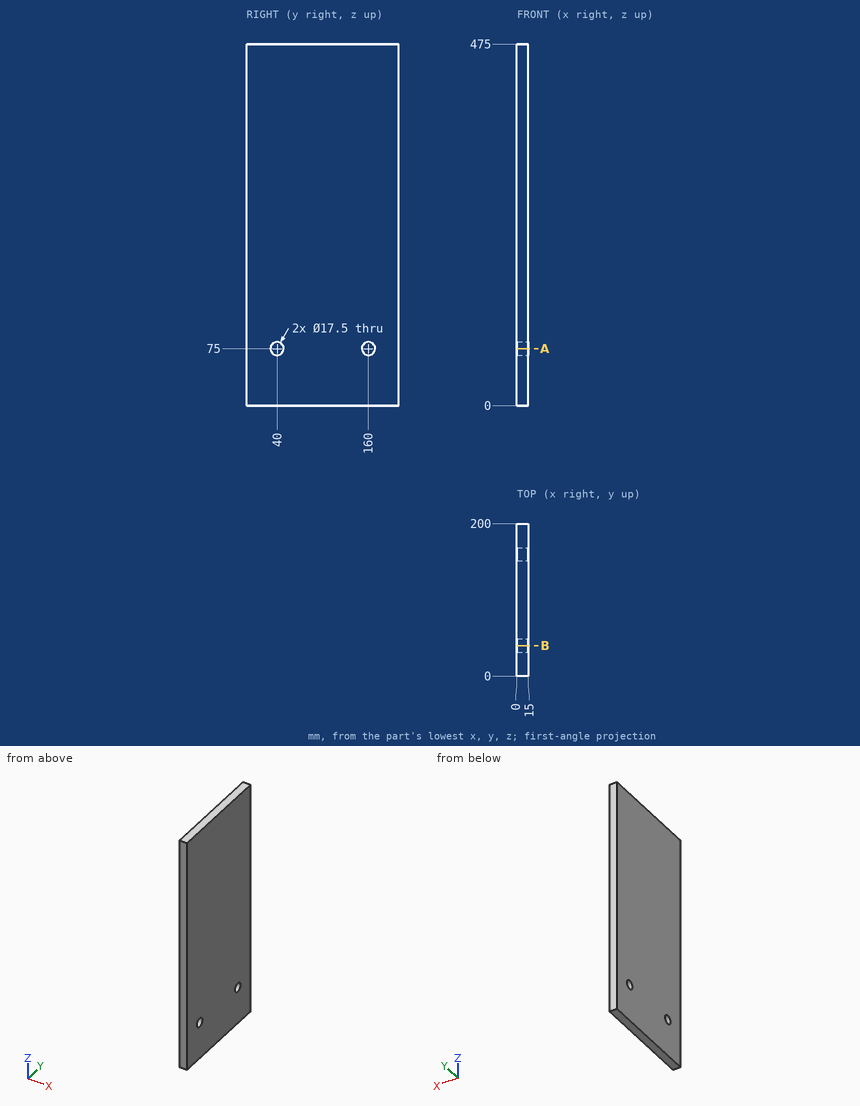
Geometry check sheet. Reference: drawing and pictorial views, mm from the part's lowest x, y, z. Give positions to 0.01 mm unless a question says otherwise; leave off trailing zeros. Write each loop counter-clockwise with the first axis right and the second up, starting at its lowest first coordinate (ties: lowest second). Pieces come first, ordered by that corner, then holes. Notation, with made-up numbers: (-11, -37.5) -> (26, -37.5) arc R11 ccw to (26, -29.5) -> close; hole circle Ø1 at (51, 74). An arc over 180 degrees is marked (long way). One line per question, with ' | ' between items.
Item 1: Sectioned sample at A-A, the plane z = 75. Record the boundary of the cut face in (x, y).
Determined:
outline: (0, 0) -> (15, 0) -> (15, 31.25) -> (0, 31.25) -> close; (0, 48.75) -> (15, 48.75) -> (15, 151.25) -> (0, 151.25) -> close; (0, 168.75) -> (15, 168.75) -> (15, 200) -> (0, 200) -> close
Item 2: Scan lines: line 1 along Z through (x, y) = (7, 160); line 2 along Y through (x, z) = (9.5, 75); line 3 along Z through (x, y) = (3.75, 32). Record each from-to range of solid material in increasing order.
Determined:
line 1: 0 to 66.25, 83.75 to 475 | line 2: 0 to 31.25, 48.75 to 151.25, 168.75 to 200 | line 3: 0 to 71.46, 78.54 to 475
Item 3: Sectioned sample at B-B, the plane y = 40. Record the boundary of the cut face in (x, z), plus the area to 3 significant figures.
Determined:
outline: (0, 0) -> (15, 0) -> (15, 66.25) -> (0, 66.25) -> close; (0, 83.75) -> (15, 83.75) -> (15, 475) -> (0, 475) -> close | area: 6,860 mm^2
